Could you check a few things on this model? Use its own coordinates, in mm. Face numbers are marked on the shaded views. A direction names the side the tool comes from. Round coordinates to 2 decimals unless told otherwise and drop trailing zeros. Loops run counter-clockwise (first coordinate to the right, second up) from the corner with the lowest first, then second, coordinate; pieces in that order, holes last. Notation, with made-up numbers: (1, 6.25) - (27, 6.25) arc R10 ccw to (27, 11.25) - close; hole circle Ø2 at (1.5, 77). An arc over 180 degrees is marked (long way). Answer as CSV lines item,"result". Start each with the question number.
1) Suppose I cut it at C-C, the plane z = 3.5. Count the separate pieces of the cut face and the enclosed holes in it, then the cut area to 3 significant figures.
2) Suppose I cut it at B-B, the plane x = 25. Write out the boundary of the cut face in (y, z).
3) I'm going to push flat-ended pins straight in: pin 1 Ø5 at (x, z) = (17, 0.5) entering from +Y; pin 2 Ø4.5 at (x, y) = (32.5, 3) entering from +Z; pin 3 Ø6 at (x, y) = (3, -7) entering from +Z. Where does each tip first touch, or does it pass through?
4) Suppose I cut it at D-D, the plane x = 5. Write out the boundary of the cut face in (y, z).
5) Suppose I cut it at A-A, the plane z = 11.25. Write out the boundary of the cut face in (x, y), then the cut area to 3 significant figures.
6) Which directions (+Z, -Z, +X, -X, +Y, -Y) give clear straight access to the entire face, cutting with the end or side of a thin tool? Please do the marked faces 1, 2, 3, 4 and 5.
7) Please list where these lines run through material, in increasing order: line 1 along Z through (x, y) = (2, -9); line 2 along Y through (x, z) = (19.5, 10.75); line 3 along Z through (x, y) = (31, -3).
```python
from build123d import *

# Parameters (mm, degrees)
SKETCH_1_W             = 26.4
SKETCH_1_H             = 34.7
SKETCH_1_R             = 1.75
EXTRUDE_1_DEPTH        = 4
EXTRUDE_1_DEPTH_BACK   = 3
EXTRUDE_START          = 4
EXTRUDE_2_DEPTH        = 6
EXTRUDE_3_DEPTH        = 1
EXTRUDE_3_DEPTH_BACK   = 3
FILLET_1_R             = 2
SKETCH_2_W             = 5
SKETCH_2_H             = 12.015250562
EXTRUDE_4_DEPTH        = 10.5
CHAMFER_2_SIZE         = 2
CHAMFER_2_SIZE2        = 3.464101615
CHAMFER_2_PART_2_SIZE  = 2
CHAMFER_2_PART_2_SIZE2 = 3.464101615
FILLET_2_R             = 0.5


with BuildPart() as part:
    # Sketch 1 → Extrude 1 (new body, two sides)
    with BuildSketch(Plane.XY) as extrude_1_sk:
        Polygon((13.064807164, 17.461834668), (13.064807164, -17.238165332), (29.24315013, -5.895849196), (21.86916953, -5.895849196), (21.86916953, 6.119401366), (29.24315013, 6.119401366), align=None)
        with Locations((-0.135192836, 0.111834668)):
            Rectangle(SKETCH_1_W, SKETCH_1_H)
        with Locations((9.85875861, -7.388165332)):
            Circle(SKETCH_1_R, mode=Mode.SUBTRACT)
        with Locations((-10.14124139, -7.388165332)):
            Circle(SKETCH_1_R, mode=Mode.SUBTRACT)
        with Locations((9.85875861, 7.611834668)):
            Circle(SKETCH_1_R, mode=Mode.SUBTRACT)
        with Locations((-10.14124139, 7.611834668)):
            Circle(SKETCH_1_R, mode=Mode.SUBTRACT)
        with BuildLine():
            Line((21.86916953, -5.895849196), (29.24315013, -5.895849196))
            ThreePointArc((29.24315013, -5.895849196), (29.53124223, 0.111776085), (29.24315013, 6.119401366))
            Line((29.24315013, 6.119401366), (21.86916953, 6.119401366))
            Line((21.86916953, 6.119401366), (21.86916953, -5.895849196))
        make_face()
        with BuildLine():
            Line((30.969143909, -5.894657137), (30.967951851, -5.895849196))
            Line((30.967951851, -5.895849196), (33.989360696, -5.895849196))
            Line((33.989360696, -5.895849196), (33.989360696, 6.119401366))
            Line((33.989360696, 6.119401366), (30.963902746, 6.119401366))
            Line((30.963902746, 6.119401366), (30.178059332, 5.333557953))
            ThreePointArc((30.178059332, 5.333557953), (30.090191367, 5.121425918), (30.178059332, 4.909293884))
            Line((30.178059332, 4.909293884), (30.757011875, 4.330341341))
            ThreePointArc((30.757011875, 4.330341341), (30.84487984, 4.118209307), (30.757011875, 3.906077273))
            Line((30.757011875, 3.906077273), (30.181275944, 3.330341341))
            ThreePointArc((30.181275944, 3.330341341), (30.093407978, 3.118209307), (30.181275944, 2.906077273))
            Line((30.181275944, 2.906077273), (30.757011875, 2.330341341))
            ThreePointArc((30.757011875, 2.330341341), (30.84487984, 2.118209307), (30.757011875, 1.906077273))
            Line((30.757011875, 1.906077273), (30.178059332, 1.32712473))
            ThreePointArc((30.178059332, 1.32712473), (30.090191367, 1.114992696), (30.178059332, 0.902860662))
            Line((30.178059332, 0.902860662), (30.757011875, 0.323908119))
            ThreePointArc((30.757011875, 0.323908119), (30.84487984, 0.111776085), (30.757011875, -0.10035595))
            Line((30.757011875, -0.10035595), (30.181275944, -0.676091881))
            ThreePointArc((30.181275944, -0.676091881), (30.093407978, -0.888223915), (30.181275944, -1.10035595))
            Line((30.181275944, -1.10035595), (30.757011875, -1.676091881))
            ThreePointArc((30.757011875, -1.676091881), (30.84487984, -1.888223915), (30.757011875, -2.10035595))
            Line((30.757011875, -2.10035595), (30.178059332, -2.679308492))
            ThreePointArc((30.178059332, -2.679308492), (30.090191367, -2.891440526), (30.178059332, -3.103572561))
            Line((30.178059332, -3.103572561), (30.757011875, -3.682525103))
            ThreePointArc((30.757011875, -3.682525103), (30.84487984, -3.894657137), (30.757011875, -4.106789172))
            Line((30.757011875, -4.106789172), (30.181275944, -4.682525103))
            ThreePointArc((30.181275944, -4.682525103), (30.093407978, -4.894657137), (30.181275944, -5.106789172))
            Line((30.181275944, -5.106789172), (30.969143909, -5.894657137))
        make_face()
    extrude(amount=EXTRUDE_1_DEPTH)
    extrude(extrude_1_sk.sketch, amount=-EXTRUDE_1_DEPTH_BACK)

    # Sketch 1_3 → Extrude 2 (add)
    with BuildSketch(Plane.XY.offset(EXTRUDE_START)):
        with BuildLine():
            Line((21.86916953, -5.895849196), (29.24315013, -5.895849196))
            ThreePointArc((29.24315013, -5.895849196), (29.53124223, 0.111776085), (29.24315013, 6.119401366))
            Line((29.24315013, 6.119401366), (21.86916953, 6.119401366))
            Line((21.86916953, 6.119401366), (21.86916953, -5.895849196))
        make_face()
        with BuildLine():
            Line((30.969143909, -5.894657137), (30.967951851, -5.895849196))
            Line((30.967951851, -5.895849196), (33.989360696, -5.895849196))
            Line((33.989360696, -5.895849196), (33.989360696, 6.119401366))
            Line((33.989360696, 6.119401366), (30.963902746, 6.119401366))
            Line((30.963902746, 6.119401366), (30.178059332, 5.333557953))
            ThreePointArc((30.178059332, 5.333557953), (30.090191367, 5.121425918), (30.178059332, 4.909293884))
            Line((30.178059332, 4.909293884), (30.757011875, 4.330341341))
            ThreePointArc((30.757011875, 4.330341341), (30.84487984, 4.118209307), (30.757011875, 3.906077273))
            Line((30.757011875, 3.906077273), (30.181275944, 3.330341341))
            ThreePointArc((30.181275944, 3.330341341), (30.093407978, 3.118209307), (30.181275944, 2.906077273))
            Line((30.181275944, 2.906077273), (30.757011875, 2.330341341))
            ThreePointArc((30.757011875, 2.330341341), (30.84487984, 2.118209307), (30.757011875, 1.906077273))
            Line((30.757011875, 1.906077273), (30.178059332, 1.32712473))
            ThreePointArc((30.178059332, 1.32712473), (30.090191367, 1.114992696), (30.178059332, 0.902860662))
            Line((30.178059332, 0.902860662), (30.757011875, 0.323908119))
            ThreePointArc((30.757011875, 0.323908119), (30.84487984, 0.111776085), (30.757011875, -0.10035595))
            Line((30.757011875, -0.10035595), (30.181275944, -0.676091881))
            ThreePointArc((30.181275944, -0.676091881), (30.093407978, -0.888223915), (30.181275944, -1.10035595))
            Line((30.181275944, -1.10035595), (30.757011875, -1.676091881))
            ThreePointArc((30.757011875, -1.676091881), (30.84487984, -1.888223915), (30.757011875, -2.10035595))
            Line((30.757011875, -2.10035595), (30.178059332, -2.679308492))
            ThreePointArc((30.178059332, -2.679308492), (30.090191367, -2.891440526), (30.178059332, -3.103572561))
            Line((30.178059332, -3.103572561), (30.757011875, -3.682525103))
            ThreePointArc((30.757011875, -3.682525103), (30.84487984, -3.894657137), (30.757011875, -4.106789172))
            Line((30.757011875, -4.106789172), (30.181275944, -4.682525103))
            ThreePointArc((30.181275944, -4.682525103), (30.093407978, -4.894657137), (30.181275944, -5.106789172))
            Line((30.181275944, -5.106789172), (30.969143909, -5.894657137))
        make_face()
    extrude(amount=EXTRUDE_2_DEPTH)

    # Sketch 1_4 → Extrude 3 (add, two sides)
    with BuildSketch(Plane.XY) as extrude_3_sk:
        with BuildLine():
            ThreePointArc((29.24315013, 6.119401366), (29.53124223, 0.111776085), (29.24315013, -5.895849196))
            Line((29.24315013, -5.895849196), (30.967951851, -5.895849196))
            Line((30.967951851, -5.895849196), (30.969143909, -5.894657137))
            Line((30.969143909, -5.894657137), (30.181275944, -5.106789172))
            ThreePointArc((30.181275944, -5.106789172), (30.093407978, -4.894657137), (30.181275944, -4.682525103))
            Line((30.181275944, -4.682525103), (30.757011875, -4.106789172))
            ThreePointArc((30.757011875, -4.106789172), (30.84487984, -3.894657137), (30.757011875, -3.682525103))
            Line((30.757011875, -3.682525103), (30.178059332, -3.103572561))
            ThreePointArc((30.178059332, -3.103572561), (30.090191367, -2.891440526), (30.178059332, -2.679308492))
            Line((30.178059332, -2.679308492), (30.757011875, -2.10035595))
            ThreePointArc((30.757011875, -2.10035595), (30.84487984, -1.888223915), (30.757011875, -1.676091881))
            Line((30.757011875, -1.676091881), (30.181275944, -1.10035595))
            ThreePointArc((30.181275944, -1.10035595), (30.093407978, -0.888223915), (30.181275944, -0.676091881))
            Line((30.181275944, -0.676091881), (30.757011875, -0.10035595))
            ThreePointArc((30.757011875, -0.10035595), (30.84487984, 0.111776085), (30.757011875, 0.323908119))
            Line((30.757011875, 0.323908119), (30.178059332, 0.902860662))
            ThreePointArc((30.178059332, 0.902860662), (30.090191367, 1.114992696), (30.178059332, 1.32712473))
            Line((30.178059332, 1.32712473), (30.757011875, 1.906077273))
            ThreePointArc((30.757011875, 1.906077273), (30.84487984, 2.118209307), (30.757011875, 2.330341341))
            Line((30.757011875, 2.330341341), (30.181275944, 2.906077273))
            ThreePointArc((30.181275944, 2.906077273), (30.093407978, 3.118209307), (30.181275944, 3.330341341))
            Line((30.181275944, 3.330341341), (30.757011875, 3.906077273))
            ThreePointArc((30.757011875, 3.906077273), (30.84487984, 4.118209307), (30.757011875, 4.330341341))
            Line((30.757011875, 4.330341341), (30.178059332, 4.909293884))
            ThreePointArc((30.178059332, 4.909293884), (30.090191367, 5.121425918), (30.178059332, 5.333557953))
            Line((30.178059332, 5.333557953), (30.963902746, 6.119401366))
            Line((30.963902746, 6.119401366), (29.24315013, 6.119401366))
        make_face()
    extrude(amount=EXTRUDE_3_DEPTH)
    extrude(extrude_3_sk.sketch, amount=-EXTRUDE_3_DEPTH_BACK)

    # Fillet 1
    fillet_1_edges = [part.edges().sort_by_distance(p)[0] for p in [
        (33.989360696, 6.119401366, 3.5),
        (33.989360696, -5.895849196, 3.5),
        (13.064807164, -17.238165332, 0.5),
        (-13.335192836, -17.238165332, 0.5),
        (-13.335192836, 17.461834668, 0.5),
        (13.064807164, 17.461834668, 0.5),
        (29.24315013, 6.119401366, -1),
        (29.24315013, -5.895849196, -1),
    ]]
    fillet(fillet_1_edges, radius=FILLET_1_R)

    # Sketch 2 → Extrude 4 (add)
    with BuildSketch(Plane.XY.offset(4)):
        with Locations((21.146996963, 0.111776085)):
            Rectangle(SKETCH_2_W, SKETCH_2_H)
    extrude(amount=EXTRUDE_4_DEPTH)

    # Chamfer 2
    chamfer_2_edges = [part.edges().sort_by_distance(p)[0] for p in [
        (21.146996963, 6.119401366, 14.5),
    ]]
    chamfer_2_side = [part.faces().sort_by_distance(p)[0] for p in [
        (23.213672797, 6.119401366, 8.3723191),
    ]]
    chamfer(chamfer_2_edges, length=CHAMFER_2_SIZE, length2=CHAMFER_2_SIZE2, reference=chamfer_2_side[0])

    # Chamfer 2 part 2
    chamfer_2_part_2_edges = [part.edges().sort_by_distance(p)[0] for p in [
        (21.146996963, -5.895849196, 14.5),
    ]]
    chamfer_2_part_2_side = [part.faces().sort_by_distance(p)[0] for p in [
        (23.213672797, -5.895849196, 8.3723191),
    ]]
    chamfer(chamfer_2_part_2_edges, length=CHAMFER_2_PART_2_SIZE, length2=CHAMFER_2_PART_2_SIZE2, reference=chamfer_2_part_2_side[0])

    # Fillet 2
    fillet_2_edges = [part.edges().sort_by_distance(p)[0] for p in [
        (23.646996963, 6.119401366, 11.25),
        (23.646996963, -5.895849196, 11.25),
        (23.646996963, 4.387350558, 13.5),
        (23.646996963, -4.163798388, 13.5),
        (18.646996963, -5.895849196, 8.25),
        (18.646996963, 6.119401366, 8.25),
        (18.646996963, 4.387350558, 13.5),
        (18.646996963, -4.163798388, 13.5),
    ]]
    fillet(fillet_2_edges, radius=FILLET_2_R)


solid = part.part
```
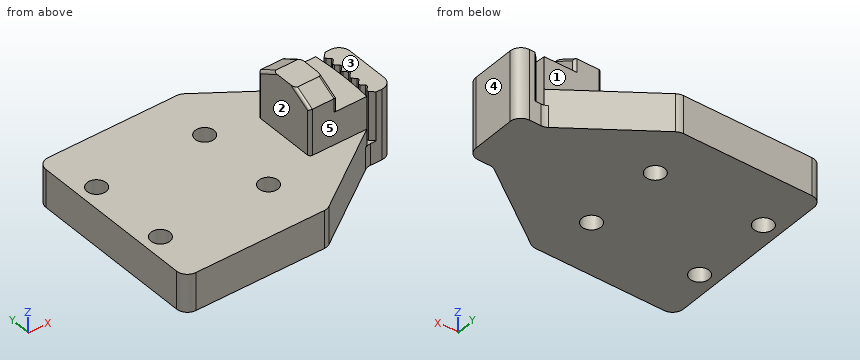
Filled sheet:
1,separate pieces,"2"
1,enclosed holes,"4"
1,area,"1,300 mm²"
2,outline,"(-8.87, -3) - (9.09, -3) - (9.09, 4) - (6.12, 4) - (6.12, 10) - (-5.9, 10) - (-5.9, 4) - (-8.87, 4) - close"
3,pin 1,"y = 16.46"
3,pin 2,"z = 10"
3,pin 3,"z = 4"
4,outline,"(-17.24, -3) - (17.46, -3) - (17.46, 4) - (-17.24, 4) - close"
5,outline,"(18.65, -5.4) arc R0.5 ccw to (19.15, -5.9) - (23.15, -5.9) arc R0.5 ccw to (23.65, -5.4) - (23.65, 5.62) arc R0.5 ccw to (23.15, 6.12) - (19.15, 6.12) arc R0.5 ccw to (18.65, 5.62) - close"
5,area,"59.9 mm²"
6,face 1,"+Z, +X, -X, +Y"
6,face 2,"+Z, -X, +Y, -Y"
6,face 3,"+Z, +X, +Y, -Y"
6,face 4,"+Z, -Z, +X, +Y, -Y"
6,face 5,"+Z, +X, -X, -Y"
7,line 1,"-3 to 4"
7,line 2,"-5.9 to 6.12"
7,line 3,"-3 to 10"
